from build123d import *

# Parameters (mm, degrees)
SKETCH_2_R          = 1.65
CUT_EXTRUDE_1_DEPTH = 23.134588318
CHAMFER_1_SIZE      = 0.8


with BuildPart() as part:
    # 草图1 → 旋转1 (revolve)
    with BuildSketch(Plane.XY, mode=Mode.PRIVATE) as revolve_1_sk:
        Polygon((0, 13.5), (11.2, 13.5), (11.2, 6.375), (14.2, 6.375), (14.2, 3.625), (7, 3.625), (7, 7.625), (0, 7.625), align=None)
    revolve(revolve_1_sk.sketch.rotate(Axis((0, 0, 0), (1, 0, 0)), 90), axis=Axis((0, 0, 0), (1, 0, 0)))

    # 草图2 → 切除-拉伸1 (cut, through all)
    with BuildSketch(Plane(origin=(11.2, 0, 0), x_dir=(0, 0, -1), z_dir=(1, 0, 0))):
        with Locations((0, 10.5)):
            Circle(SKETCH_2_R)
        with Locations((10.5, 0)):
            Circle(SKETCH_2_R)
        with Locations((0, -10.5)):
            Circle(SKETCH_2_R)
        with Locations((-10.5, 0)):
            Circle(SKETCH_2_R)
    extrude(amount=-CUT_EXTRUDE_1_DEPTH, mode=Mode.SUBTRACT)

    # 倒角1
    chamfer_1_edges = [part.edges().sort_by_distance(p)[0] for p in [
        (0, 0, -7.625),
        (0, 0, -13.5),
        (11.2, 0, -13.5),
        (14.2, 0, -6.375),
    ]]
    chamfer(chamfer_1_edges, length=CHAMFER_1_SIZE)


solid = part.part
Geometry: final body of the model. Coordinates: model frame, mm. A direction names the side the tool comes from. Give positions to 0.01 mm unless a question says otherwise; leave off trailing zeros. Order: outer loops, then holes, each group sorted by start corner. A loop starts at its lowest first (then second) coordinate and runs counter-clockwise, first axis right, second up. Notation, with made-up numbers: (61.25, 59) -> (102.25, 59) arc R13 ccw to (102.25, 81) -> close; hole circle Ø6 at (66.25, -40). An arc over 180 degrees is marked (long way). Answer as a JSON object with one key per item and string values.
Q1. Section C-C (x = 6). Output: boundary loops of the cut face in (y, z) (3 decimals).
Entries:
{"outline": "circle Ø27 at (0, 0); hole circle Ø3.3 at (-10.5, 0); hole circle Ø15.25 at (0, 0); hole circle Ø3.3 at (0, -10.5); hole circle Ø3.3 at (0, 10.5); hole circle Ø3.3 at (10.5, 0)"}
Q2. First-contact query: pin 1 (4.5 mm diameter, centred on y = 0, z = 0, fed in from +X); pin 2 (5.5 mm diameter, centred on y = 10.5, z = 0, fed in from +X); pin 3 (6 mm diameter, centred on x = 7, z = -6.5, fed in from +Y); pin 4 (1.5 mm diameter, centred on x = 3, z = -9.5, fed in from +Y). Flat tips, straight axial feed; report the tip coordinate or a pass-through.
Entries:
{"pin 1": "passes through", "pin 2": "stops at x = 11.2", "pin 3": "stops at y = 13.04", "pin 4": "stops at y = 10.28"}
Q3. Section D-D (x = 12.5). Output: boundary loops of the cut face in (y, z) (3 decimals).
Entries:
{"outline": "circle Ø12.75 at (0, 0); hole circle Ø7.25 at (0, 0)"}
Q4. Material intervals for probe 1 along Y at (x, z) = (9.25, 0) (3 decimals); probe 2 along Y at (x, z) = (6.75, 0) (3 decimals); probe 3 along Z at (x, y) = (2.5, -0.75), sorted ascending.
Entries:
{"probe 1": "y = -13.5 to -12.15, -8.85 to -3.625, 3.625 to 8.85, 12.15 to 13.5", "probe 2": "y = -13.5 to -12.15, -8.85 to -7.625, 7.625 to 8.85, 12.15 to 13.5", "probe 3": "z = -13.48 to -11.97, -9.03 to -7.59, 7.59 to 9.03, 11.97 to 13.48"}
Q5. Access query for faces 4 (the cylindrical face through (5.7, 8.9, 0.4)), 5 (the cylindrical face through (3.857, 7.444, -1.653)). Directions: +Z, -Z, +X, -X, +Y, -Y. A direction counts if a zero-diameter tool reaches every point of the face in a straight line with its end or side. Return the directions, or none.
Entries:
{"face 4": "+X, -X", "face 5": "-X"}
Q6. Section A-A (y = 0). State how many separate pieces and enclosed holes the cut face has, plus the area to 3 significant figures.
Entries:
{"separate pieces": "4", "enclosed holes": "0", "area": "105 mm^2"}
Q7. Draft query along Z for faces 1 (the cylindrical face through (5.7, -12.1, 0.4)), 2 (the cylindrical face through (12.32, 3.88, -5.06)), 3 (the flat face through (11.2, 3, -6)). Return one class per face: released by +Z, released by -Z, zero draft, split by the parting line, or undercut.
Entries:
{"face 1": "undercut", "face 2": "split by the parting line", "face 3": "zero draft"}
